from build123d import *

# Parameters (mm, degrees)
SKETCH1_W                                    = 80
SKETCH1_H                                    = 56
BOSS_EXTRUDE1_DEPTH                          = 3
SKETCH2_W                                    = 74
SKETCH2_H                                    = 50
BOSS_EXTRUDE2_DEPTH                          = 24
FILLET1_R                                    = 1
FILLET2_R                                    = 2
SKETCH3_R                                    = 2.5
CUT_EXTRUDE1_DEPTH                           = 10
CUT_EXTRUDE2_DEPTH                           = 10
FILLET3_R                                    = 2
BOSS_EXTRUDE3_DEPTH                          = 2
CUT_EXTRUDE3_DEPTH                           = 89.090862182
CBORE_FOR_M3_CROSS_RECESS_PAN_HEAD_S_2_COUNT = 2
CBORE_FOR_M3_CROSS_RECESS_PAN_HEAD_S_2_PITCH = 15.207328374
CBORE_FOR_M3_CROSS_RECESS_PAN_HEAD_S_3_COUNT = 2
CBORE_FOR_M3_CROSS_RECESS_PAN_HEAD_S_3_PITCH = 14.900401376


with BuildPart() as part:
    # Sketch1 → Boss-Extrude1 (new body)
    with BuildSketch(Plane(origin=(0, 0, 0), x_dir=(1, 0, 0), z_dir=(0, 1, 0))):
        Rectangle(SKETCH1_W, SKETCH1_H)
    extrude(amount=BOSS_EXTRUDE1_DEPTH)

    # Sketch2 → Boss-Extrude2 (add)
    with BuildSketch(Plane.XZ):
        Polygon((37, -28), (-37, -28), (-40, -28), (-40, 28), (40, 28), (40, -28), align=None)
        Rectangle(SKETCH2_W, SKETCH2_H, mode=Mode.SUBTRACT)
    extrude(amount=BOSS_EXTRUDE2_DEPTH)

    # Fillet1
    fillet1_edges = [part.edges().sort_by_distance(p)[0] for p in [
        (-37, -12, -25),
        (37, -12, -25),
        (37, -12, 25),
        (-37, -12, 25),
    ]]
    fillet(fillet1_edges, radius=FILLET1_R)

    # Fillet2
    fillet2_edges = [part.edges().sort_by_distance(p)[0] for p in [
        (-40, 3, 0),
        (0, 3, 28),
        (40, 3, 0),
        (40, -10.5, 28),
        (-40, -10.5, 28),
        (-40, -10.5, -28),
        (40, -10.5, -28),
        (0, 3, -28),
    ]]
    fillet(fillet2_edges, radius=FILLET2_R)

    # Sketch3 → Cut-Extrude1 (cut)
    with BuildSketch(Plane.XY.offset(28)):
        with Locations((0, -16.5)):
            Circle(SKETCH3_R)
        with Locations((-20, -16.5)):
            Circle(SKETCH3_R)
        with Locations(Location((20, -16.5, 0), (0, 0, 180))):
            Circle(SKETCH3_R)
    extrude(amount=-CUT_EXTRUDE1_DEPTH, mode=Mode.SUBTRACT)

    # Sketch5 → Cut-Extrude2 (cut)
    with BuildSketch(Plane(origin=(0, 0, -28), x_dir=(-1, 0, 0), z_dir=(0, 0, -1))):
        with BuildLine():
            Line((-27, -1), (-23, -1))
            ThreePointArc((-23, -1), (-20, -4), (-23, -7))
            Line((-23, -7), (-27, -7))
            ThreePointArc((-27, -7), (-30, -4), (-27, -1))
        make_face()
    extrude(amount=-CUT_EXTRUDE2_DEPTH, mode=Mode.SUBTRACT)

    # Fillet3
    fillet3_edges = [part.edges().sort_by_distance(p)[0] for p in [
        (30, -4, -28),
        (25, -7, -28),
        (20, -4, -28),
        (25, -1, -28),
    ]]
    fillet(fillet3_edges, radius=FILLET3_R - 0.0001)  # a hair under: the kernel refuses the full size

    # Sketch6 → Boss-Extrude3 (add)
    with BuildSketch(Plane.XZ):
        with BuildLine():
            Line((37, 18.5), (33, 18.5))
            ThreePointArc((33, 18.5), (31.232233047, 19.232233047), (30.5, 21))
            Line((30.5, 21), (30.5, 25))
            Line((30.5, 25), (37, 25))
            Line((37, 25), (37, 18.5))
        make_face()
        with BuildLine():
            Line((37, -5), (30.5, -5))
            Line((30.5, -5), (30.5, -1))
            ThreePointArc((30.5, -1), (31.232233047, 0.767766953), (33, 1.5))
            Line((33, 1.5), (37, 1.5))
            Line((37, 1.5), (37, -5))
        make_face()
        with BuildLine():
            Line((-29, 1.5), (-25, 1.5))
            ThreePointArc((-25, 1.5), (-23.232233047, 0.767766953), (-22.5, -1))
            Line((-22.5, -1), (-22.5, -5))
            Line((-22.5, -5), (-29, -5))
            Line((-29, -5), (-29, 1.5))
        make_face()
        with BuildLine():
            Line((-29, 25), (-22.5, 25))
            Line((-22.5, 25), (-22.5, 21))
            ThreePointArc((-22.5, 21), (-23.232233047, 19.232233047), (-25, 18.5))
            Line((-25, 18.5), (-29, 18.5))
            Line((-29, 18.5), (-29, 25))
        make_face()
    extrude(amount=BOSS_EXTRUDE3_DEPTH)

    # Sketch7 → Cut-Extrude3 (cut, through all)
    with BuildSketch(Plane.ZY.offset(40)):
        with BuildLine():
            Line((-16.5, -6.5), (-16.5, -16.5))
            ThreePointArc((-16.5, -16.5), (-17.5, -17.5), (-18.5, -16.5))
            Line((-18.5, -16.5), (-18.5, -6.5))
            ThreePointArc((-18.5, -6.5), (-17.5, -5.5), (-16.5, -6.5))
        make_face()
        with BuildLine():
            Line((-11.5, -6.5), (-11.5, -16.5))
            ThreePointArc((-11.5, -16.5), (-12.5, -17.5), (-13.5, -16.5))
            Line((-13.5, -16.5), (-13.5, -6.5))
            ThreePointArc((-13.5, -6.5), (-12.5, -5.5), (-11.5, -6.5))
        make_face()
        with BuildLine():
            Line((-6.5, -6.5), (-6.5, -16.5))
            ThreePointArc((-6.5, -16.5), (-7.5, -17.5), (-8.5, -16.5))
            Line((-8.5, -16.5), (-8.5, -6.5))
            ThreePointArc((-8.5, -6.5), (-7.5, -5.5), (-6.5, -6.5))
        make_face()
        with BuildLine():
            Line((-1.5, -6.5), (-1.5, -16.5))
            ThreePointArc((-1.5, -16.5), (-2.5, -17.5), (-3.5, -16.5))
            Line((-3.5, -16.5), (-3.5, -6.5))
            ThreePointArc((-3.5, -6.5), (-2.5, -5.5), (-1.5, -6.5))
        make_face()
        with BuildLine():
            Line((3.5, -6.5), (3.5, -16.5))
            ThreePointArc((3.5, -16.5), (2.5, -17.5), (1.5, -16.5))
            Line((1.5, -16.5), (1.5, -6.5))
            ThreePointArc((1.5, -6.5), (2.5, -5.5), (3.5, -6.5))
        make_face()
        with BuildLine():
            Line((8.5, -6.5), (8.5, -16.5))
            ThreePointArc((8.5, -16.5), (7.5, -17.5), (6.5, -16.5))
            Line((6.5, -16.5), (6.5, -6.5))
            ThreePointArc((6.5, -6.5), (7.5, -5.5), (8.5, -6.5))
        make_face()
        with BuildLine():
            Line((13.5, -6.5), (13.5, -16.5))
            ThreePointArc((13.5, -16.5), (12.5, -17.5), (11.5, -16.5))
            Line((11.5, -16.5), (11.5, -6.5))
            ThreePointArc((11.5, -6.5), (12.5, -5.5), (13.5, -6.5))
        make_face()
        with BuildLine():
            Line((18.5, -6.5), (18.5, -16.5))
            ThreePointArc((18.5, -16.5), (17.5, -17.5), (16.5, -16.5))
            Line((16.5, -16.5), (16.5, -6.5))
            ThreePointArc((16.5, -6.5), (17.5, -5.5), (18.5, -6.5))
        make_face()
    extrude(amount=-CUT_EXTRUDE3_DEPTH, mode=Mode.SUBTRACT)

    # Sketch9 → CBORE for M3 Cross Recess Pan Head Screw1 (revolve, cut)
    with BuildSketch(Plane(origin=(40, -21, -20.8), x_dir=(0, 0, -1), z_dir=(0, 1, 0))):
        Polygon((0, 0), (0, 3), (1.7, 3), (1.7, 2.4), (2.5, 2.4), (2.5, 0), align=None)
    cbore_for_m3_cross_recess_pan_head_screw = revolve(axis=Axis((46.35, -21, -20.8), (-1, 0, 0)), mode=Mode.SUBTRACT)

    # CBORE for M3 Cross Recess Pan Head S 2: CBORE for M3 Cross Recess Pan Head Screw1 ×2
    with Locations(*[Vector(0, -0.1073379095741248, -0.9942225973936909) * (i * CBORE_FOR_M3_CROSS_RECESS_PAN_HEAD_S_2_PITCH) for i in range(1, CBORE_FOR_M3_CROSS_RECESS_PAN_HEAD_S_2_COUNT)]):
        add(cbore_for_m3_cross_recess_pan_head_screw, mode=Mode.SUBTRACT)

    # CBORE for M3 Cross Recess Pan Head S 3: CBORE for M3 Cross Recess Pan Head Screw1 ×2
    with Locations(*[Vector(0, -0.0825685481728506, -0.9965853876375209) * (i * CBORE_FOR_M3_CROSS_RECESS_PAN_HEAD_S_3_PITCH) for i in range(1, CBORE_FOR_M3_CROSS_RECESS_PAN_HEAD_S_3_COUNT)]):
        add(cbore_for_m3_cross_recess_pan_head_screw, mode=Mode.SUBTRACT)

    # Mirror1: CBORE for M3 Cross Recess Pan Head Screw1 across plane
    add(cbore_for_m3_cross_recess_pan_head_screw.mirror(Plane.XY), mode=Mode.SUBTRACT)

    # Mirror1 copy 1 sketch → Mirror1 copy 1 (revolve, cut)
    with BuildSketch(Plane(origin=(40, -22.632322838, 35.919469515), x_dir=(0, 0, 1), z_dir=(0, 1, 0))):
        Polygon((0, 0), (0, -3), (1.7, -3), (1.7, -2.4), (2.5, -2.4), (2.5, 0), align=None)
    revolve(axis=Axis((46.35, -22.632322838, 35.919469515), (1, 0, 0)), mode=Mode.SUBTRACT)

    # Mirror1 copy 2 sketch → Mirror1 copy 2 (revolve, cut)
    with BuildSketch(Plane(origin=(40, -22.230304509, 35.649522281), x_dir=(0, 0, 1), z_dir=(0, 1, 0))):
        Polygon((0, 0), (0, -3), (1.7, -3), (1.7, -2.4), (2.5, -2.4), (2.5, 0), align=None)
    revolve(axis=Axis((46.35, -22.230304509, 35.649522281), (1, 0, 0)), mode=Mode.SUBTRACT)

    # Mirror2: CBORE for M3 Cross Recess Pan Head Screw1 across plane
    add(cbore_for_m3_cross_recess_pan_head_screw.mirror(Plane(origin=(0, 0, 0), x_dir=(0, 0, 1), z_dir=(1, 0, 0))), mode=Mode.SUBTRACT)

    # Mirror2 copy 1 sketch → Mirror2 copy 1 (revolve, cut)
    with BuildSketch(Plane(origin=(-40, -22.632322838, -35.919469515), x_dir=(0, 0, -1), z_dir=(0, 1, 0))):
        Polygon((0, 0), (0, -3), (1.7, -3), (1.7, -2.4), (2.5, -2.4), (2.5, 0), align=None)
    revolve(axis=Axis((-46.35, -22.632322838, -35.919469515), (-1, 0, 0)), mode=Mode.SUBTRACT)

    # Mirror2 copy 2 sketch → Mirror2 copy 2 (revolve, cut)
    with BuildSketch(Plane(origin=(-40, -22.230304509, -35.649522281), x_dir=(0, 0, -1), z_dir=(0, 1, 0))):
        Polygon((0, 0), (0, -3), (1.7, -3), (1.7, -2.4), (2.5, -2.4), (2.5, 0), align=None)
    revolve(axis=Axis((-46.35, -22.230304509, -35.649522281), (-1, 0, 0)), mode=Mode.SUBTRACT)

    # Mirror2 copy 3 sketch → Mirror2 copy 3 (revolve, cut)
    with BuildSketch(Plane(origin=(-40, -21, 20.8), x_dir=(0, 0, 1), z_dir=(0, 1, 0))):
        Polygon((0, 0), (0, 3), (1.7, 3), (1.7, 2.4), (2.5, 2.4), (2.5, 0), align=None)
    revolve(axis=Axis((-46.35, -21, 20.8), (1, 0, 0)), mode=Mode.SUBTRACT)

    # Mirror2 copy 4 sketch → Mirror2 copy 4 (revolve, cut)
    with BuildSketch(Plane(origin=(-40, -22.632322838, 35.919469515), x_dir=(0, 0, 1), z_dir=(0, 1, 0))):
        Polygon((0, 0), (0, 3), (1.7, 3), (1.7, 2.4), (2.5, 2.4), (2.5, 0), align=None)
    revolve(axis=Axis((-46.35, -22.632322838, 35.919469515), (1, 0, 0)), mode=Mode.SUBTRACT)

    # Mirror2 copy 5 sketch → Mirror2 copy 5 (revolve, cut)
    with BuildSketch(Plane(origin=(-40, -22.230304509, 35.649522281), x_dir=(0, 0, 1), z_dir=(0, 1, 0))):
        Polygon((0, 0), (0, 3), (1.7, 3), (1.7, 2.4), (2.5, 2.4), (2.5, 0), align=None)
    revolve(axis=Axis((-46.35, -22.230304509, 35.649522281), (1, 0, 0)), mode=Mode.SUBTRACT)


solid = part.part
Could you check a few things on this model? Use its own coordinates, in mm. A direction names the side the tool comes from. Round coordinates to 2 decimals unless told otherwise and drop trailing zeros. Write each loop counter-clockwise with the first axis right and the second up, starting at its lowest first coordinate (ties: lowest second). Pieces come first, ordered by that corner, then holes. Notation, with made-up numbers: (-39.5, -6.75) - (4.5, -6.75) arc R28 ccw to (4.5, 28.25) - close; hole circle Ø10 at (41, -17). An arc over 180 degrees is marked (long way). Use a Markdown table: item, result.
Q1. For pin 1 (3 mm diameter, centred on x = 33.5, z = 23, fed in from -Y); pin 2 (3 mm diameter, centred on x = -29, z = 12, fed in from -Y), each with a flat end and sliding along its axis, tell me the tip position at first contact or that it passes through.
Output values:
| item | result |
|---|---|
| pin 1 | y = -2 |
| pin 2 | y = 0 |
Q2. For faces 1 (the flat face through (38, -11, 13.5)), 2 (the cylindrical face through (31.252, -0.986, 19.213)), 3 (the cylindrical face through (20, -3.9, -25.5)), which set-ups out of +Z, -Z, +X, -X, +Y, -Y let a thin tool reach every point of the face, with its end or its side?
Output values:
| item | result |
|---|---|
| face 1 | +X, -X |
| face 2 | -Y |
| face 3 | -Z |
Q3. I want a section at C-C (y = -21). Count the separate pieces of the cut face and the enclosed holes in it, plus the area to 3 significant figures.
Output values:
| item | result |
|---|---|
| separate pieces | 4 |
| enclosed holes | 0 |
| area | 721 mm2 |
Q4. I want a section at B-B (z = 12.5). List the corners of the cut face in (x, y) for me.
Output values:
| item | result |
|---|---|
| outline | (-40, -24) - (-37, -24) - (-37, -17.5) - (-40, -17.5) - close; (-40, -5.5) - (-37, -5.5) - (-37, 0) - (37, 0) - (37, -5.5) - (40, -5.5) - (40, 1) arc R2 ccw to (38, 3) - (-38, 3) arc R2 ccw to (-40, 1) - close; (37, -24) - (40, -24) - (40, -17.5) - (37, -17.5) - close |
Q5. Please list where these lines run through material, in increasing order: L1, parallel to Z at x = -37.5, y = -21; L2, parallel to X at y = -10, z = -21.5; L3, parallel to Z at x = 5.5, y = -12.
Output values:
| item | result |
|---|---|
| L1 | -28 to -22.5, -19.1 to 19.1, 22.5 to 28 |
| L2 | -40 to -37, 37 to 40 |
| L3 | -28 to -25, 25 to 28 |
Q6. I want a section at D-D (z = 5.5). List the corners of the cut face in (x, y) for me.
Output values:
| item | result |
|---|---|
| outline | (-40, -24) - (-37, -24) - (-37, 0) - (37, 0) - (37, -24) - (40, -24) - (40, 1) arc R2 ccw to (38, 3) - (-38, 3) arc R2 ccw to (-40, 1) - close |
Q7. Thinking about a two-plate mould opening in Z: for faces 4 (the cylindrical face through (0.53, 2.4, 27.43)), 5 (the cylindrical face through (39.43, 2.4, -0.36)), 6 (the flat face through (-26, -1, -5)), 7 (the cylindrical face through (-39.4, -11.32, -27.43)), which applies, released by +Z, released by -Z, zero draft, split by the parting line, or undercut?
Output values:
| item | result |
|---|---|
| face 4 | released by +Z |
| face 5 | zero draft |
| face 6 | undercut |
| face 7 | released by -Z |
Q8. I want a section at A-A (x = -20). List the corners of the cut face in (y, z) for me, plus the area to 3 significant figures.
Output values:
| item | result |
|---|---|
| outline | (-24, -28) - (1, -28) arc R2 ccw to (3, -26) - (3, 26) arc R2 ccw to (1, 28) - (-14, 28) - (-14, 25) - (0, 25) - (0, -25) - (-24, -25) - close; (-24, 25) - (-19, 25) - (-19, 28) - (-24, 28) - close |
| area | 295 mm2 |
